```python
from build123d import *

# Parameters (mm, degrees)
SKETCH_1_R      = 1.6
EXTRUDE_1_DEPTH = 3


with BuildPart() as part:
    # 草图1 → 凸台-拉伸1 (new body)
    with BuildSketch(Plane(origin=(0, 0, 0), x_dir=(1, 0, 0), z_dir=(0, 1, 0))):
        with BuildLine():
            Line((-31.220966692, 4), (-36.292034504, -1.071067812))
            ThreePointArc((-36.292034504, -1.071067812), (-39.536267992, -3.238795325), (-43.363102316, -4))
            Line((-43.363102316, -4), (-46.95, -4))
            Line((-46.95, -4), (-83.804594146, -4))
            Line((-83.804594146, -4), (-93.814764296, -4))
            ThreePointArc((-93.814764296, -4), (0, 93.9), (93.814764296, -4))
            Line((93.814764296, -4), (83.804594146, -4))
            Line((83.804594146, -4), (46.95, -4))
            Line((46.95, -4), (43.363102316, -4))
            ThreePointArc((43.363102316, -4), (39.536267992, -3.238795325), (36.292034504, -1.071067812))
            Line((36.292034504, -1.071067812), (31.220966692, 4))
            Line((31.220966692, 4), (4, 31.220966692))
            ThreePointArc((4, 31.220966692), (0, 32.877820942), (-4, 31.220966692))
            Line((-4, 31.220966692), (-31.220966692, 4))
        make_face()
        with Locations(Location((88.9, 0, 0), (0, 0, 270))):
            Circle(SKETCH_1_R, mode=Mode.SUBTRACT)
        with Locations(Location((-88.9, 0, 0), (0, 0, 270))):
            Circle(SKETCH_1_R, mode=Mode.SUBTRACT)
        with Locations(Location((-62.861792847, 62.861792847, 0), (0, 0, 270))):
            Circle(SKETCH_1_R, mode=Mode.SUBTRACT)
        with Locations(Location((0, 88.9, 0), (0, 0, 270))):
            Circle(SKETCH_1_R, mode=Mode.SUBTRACT)
        with Locations(Location((62.861792847, 62.861792847, 0), (0, 0, 270))):
            Circle(SKETCH_1_R, mode=Mode.SUBTRACT)
        with BuildLine():
            Line((46.95, 4), (47.760369555, 4))
            ThreePointArc((47.760369555, 4), (55.764412134, 8.005393892), (57.356586062, 16.812939522))
            ThreePointArc((57.356586062, 16.812939522), (42.263772312, 42.263772312), (16.812939522, 57.356586062))
            ThreePointArc((16.812939522, 57.356586062), (8.005393892, 55.764412134), (4, 47.760369555))
            Line((4, 47.760369555), (4, 46.95))
            Line((4, 46.95), (4, 41.363102316))
            ThreePointArc((4, 41.363102316), (4.761204675, 37.536267992), (6.928932188, 34.292034504))
            Line((6.928932188, 34.292034504), (34.292034504, 6.928932188))
            ThreePointArc((34.292034504, 6.928932188), (37.536267992, 4.761204675), (41.363102316, 4))
            Line((41.363102316, 4), (46.95, 4))
        make_face(mode=Mode.SUBTRACT)
        with BuildLine():
            Line((-46.95, 4), (-41.363102316, 4))
            ThreePointArc((-41.363102316, 4), (-37.536267992, 4.761204675), (-34.292034504, 6.928932188))
            Line((-34.292034504, 6.928932188), (-6.928932188, 34.292034504))
            ThreePointArc((-6.928932188, 34.292034504), (-4.761204675, 37.536267992), (-4, 41.363102316))
            Line((-4, 41.363102316), (-4, 46.95))
            Line((-4, 46.95), (-4, 47.760369555))
            ThreePointArc((-4, 47.760369555), (-8.005393892, 55.764412134), (-16.812939522, 57.356586062))
            ThreePointArc((-16.812939522, 57.356586062), (-42.263772312, 42.263772312), (-57.356586062, 16.812939522))
            ThreePointArc((-57.356586062, 16.812939522), (-55.764412134, 8.005393892), (-47.760369555, 4))
            Line((-47.760369555, 4), (-46.95, 4))
        make_face(mode=Mode.SUBTRACT)
        with BuildLine():
            Line((-78.53185914, 4), (-81.679924094, 4))
            ThreePointArc((-81.679924094, 4), (-83.145024823, 4.638574331), (-83.674549835, 6.146520147))
            ThreePointArc((-83.674549835, 6.146520147), (-59.326258942, 59.326258942), (-6.146520147, 83.674549835))
            ThreePointArc((-6.146520147, 83.674549835), (-4.638574331, 83.145024823), (-4, 81.679924094))
            Line((-4, 81.679924094), (-4, 78.53185914))
            ThreePointArc((-4, 78.53185914), (-6.333499574, 72.111207209), (-12.244954243, 68.687072987))
            ThreePointArc((-12.244954243, 68.687072987), (-49.334840123, 49.334840123), (-68.687072987, 12.244954243))
            ThreePointArc((-68.687072987, 12.244954243), (-72.111207209, 6.333499574), (-78.53185914, 4))
        make_face(mode=Mode.SUBTRACT)
        with BuildLine():
            Line((4, 78.53185914), (4, 81.679924094))
            ThreePointArc((4, 81.679924094), (4.638574331, 83.145024823), (6.146520147, 83.674549835))
            ThreePointArc((6.146520147, 83.674549835), (59.326258942, 59.326258942), (83.674549835, 6.146520147))
            ThreePointArc((83.674549835, 6.146520147), (83.145024823, 4.638574331), (81.679924094, 4))
            Line((81.679924094, 4), (78.53185914, 4))
            ThreePointArc((78.53185914, 4), (72.111207209, 6.333499574), (68.687072987, 12.244954243))
            ThreePointArc((68.687072987, 12.244954243), (49.334840123, 49.334840123), (12.244954243, 68.687072987))
            ThreePointArc((12.244954243, 68.687072987), (6.333499574, 72.111207209), (4, 78.53185914))
        make_face(mode=Mode.SUBTRACT)
    extrude(amount=EXTRUDE_1_DEPTH)


solid = part.part
```
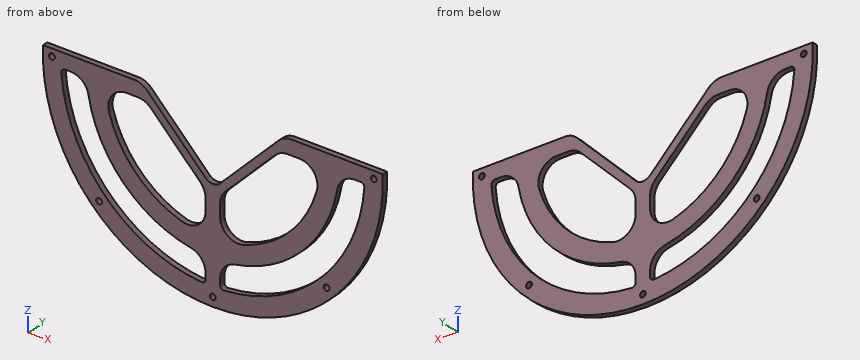
The listing builds one solid part. Answer for the finished solid, in the listing's coordinates (mm). Coordinates: 2 decimals unless noted, no trailing zeros. Loops run counter-clockwise (first coordinate to the right, second up) from the corner with the lowest first, then second, coordinate; pieces in that order, holes last. Notation, with made-up numbers: M 12.5,56 L 19.5,56 A18 cw 19.5,79 Z; hole C -10.75,-14.5 d4. An arc over 180 degrees is marked long. Answer as a JSON object with one key per item and string values. Group by question number.
Item 1: Each of these flat-tipped pins is pushed along its axis until it touches: P1, Ø1.5, axis at x = 44.5, y = 2, coming from the -Z side; P2, Ø5, axis at x = -62.86, z = -62.86, coming from the -Y side; P3, Ø1.5, axis at y = 1, z = -79.5, coming from the +X side; P4, Ø0.9, axis at x = -44.5, y = 1.5, coming from the -Z side. Where does it stop, or does it pass through?
Item 2: Section C-C (x = -55) is taken. Write down the section's boundary in (y, z).
Item 3: Consider L1, parallel to Z at x = 10.5, y = 0.2; L2, parallel to X at y = 2.5, z = -14; L3, parallel to X at y = 1.8, z = 0. Determine where each line is inside the solid, lowest interval first.
Item 4: Section A-A (x = 9.5) is taken. Write down the section's boundary in (y, z), and give its area (3 significant figures).
Item 5: Section D-D (y = 1.3) is taken. Give the number of separate pieces and of enclosed holes in the cut face, and give its area (3 significant figures).
Item 6: Section B-B (z = -14) is taken. Write down the section's boundary in (x, y), and give its area (3 significant figures).
Solved:
{
 "1": {"P1": "stops at z = -83.09", "P2": "stops at y = 0", "P3": "stops at x = 51.14", "P4": "stops at z = -82.93"},
 "2": {"outline": "M 0,-76.11 L 3,-76.11 L 3,-63.36 L 0,-63.36 Z; M 0,-42.93 L 3,-42.93 L 3,-23.4 L 0,-23.4 Z; M 0,-7.1 L 3,-7.1 L 3,4 L 0,4 Z"},
 "3": {"L1": "z = -93.31 to -83.24, -69.16 to -57.13, -30.72 to -24.72", "L2": "x = -92.85 to -82.72, -68.35 to -57.76, -27.22 to -21.22, 21.22 to 27.22, 57.76 to 68.35, 82.72 to 92.85", "L3": "x = -93.9 to -90.5, -87.3 to -35.22, 35.22 to 87.3, 90.5 to 93.9"},
 "4": {"outline": "M 0,-93.42 L 3,-93.42 L 3,-83.36 L 0,-83.36 Z; M 0,-69.6 L 3,-69.6 L 3,-56.69 L 0,-56.69 Z; M 0,-31.72 L 3,-31.72 L 3,-25.72 L 0,-25.72 Z", "area": "86.9 mm2"},
 "5": {"separate pieces": "1", "enclosed holes": "9", "area": "6,470 mm2"},
 "6": {"outline": "M -92.85,0 L -82.72,0 L -82.72,3 L -92.85,3 Z; M -68.35,0 L -57.76,0 L -57.76,3 L -68.35,3 Z; M -27.22,0 L -21.22,0 L -21.22,3 L -27.22,3 Z; M 21.22,0 L 27.22,0 L 27.22,3 L 21.22,3 Z; M 57.76,0 L 68.35,0 L 68.35,3 L 57.76,3 Z; M 82.72,0 L 92.85,0 L 92.85,3 L 82.72,3 Z", "area": "160 mm2"}
}
